```python
from build123d import *

# Parameters (mm, degrees)
F0_W      = 30
F0_H      = 50
F1_DEPTH  = 400
F3_D      = 20
F4_DEPTH  = 4.6
F5_W      = 10
F5_H      = 50
F6_DEPTH  = 20
F7_W      = 10
F7_H      = 25
F9_W      = 10
F9_H      = 25
F12_D     = 20
F13_W     = 30
F13_H     = 100
F14_DEPTH = 50
F16_D     = 10


with BuildPart() as f1:
    # F0 (on Front) → F1 (new body)
    with BuildSketch(Plane.XZ):
        with Locations((15, 25)):
            Rectangle(F0_W, F0_H)
    extrude(amount=F1_DEPTH)

    # F3 (through all)
    with Locations(Plane(origin=(0, 0, 0), x_dir=(0, 1, 0), z_dir=(-1, 0, 0))):
        with Locations((-375, -25), (-57.4, -25)):
            Hole(F3_D / 2)

    # F0 (on Front) → F4 (join)
    with BuildSketch(Plane.XZ):
        with Locations((15, 25)):
            Rectangle(F0_W, F0_H)
    extrude(amount=-F4_DEPTH)

    # F5 (on Right) → F6 (join)
    with BuildSketch(Plane.YZ):
        with Locations((-0.4, 25)):
            Rectangle(F5_W, F5_H)
        with Locations((-114.4, 25)):
            Rectangle(F5_W, F5_H)
    extrude(amount=-F6_DEPTH)

    # F7 (on face) → F8 (revolve)
    with BuildSketch(Plane(origin=(-20, 0, 0), x_dir=(0, -1, 0), z_dir=(-1, 0, 0))):
        with Locations((0.4, 12.5)):
            Rectangle(F7_W, F7_H)
    revolve(axis=Axis((-20, -0.4124408588, 25), (0, -1, 0)))

    # F9 (on face) → F10 (revolve)
    with BuildSketch(Plane(origin=(-20, 0, 0), x_dir=(0, -1, 0), z_dir=(-1, 0, 0))):
        with Locations((114.4, 12.5)):
            Rectangle(F9_W, F9_H)
    revolve(axis=Axis((-20, -114.0791960061, 25), (0, -1, 0)))

    # F12 (through all)
    with Locations(Plane(origin=(0, 4.6, 0), x_dir=(-1, 0, 0), z_dir=(0, 1, 0))):
        with Locations((20, 25)):
            Hole(F12_D / 2)

    # F13 (on face) → F14 (join)
    with BuildSketch(Plane(origin=(0, 0, 0), x_dir=(1, 0, 0), z_dir=(0, 0, -1))):
        with Locations((15, 57.4)):
            Rectangle(F13_W, F13_H)
    extrude(amount=F14_DEPTH)

    # F16 (through all)
    with Locations(Plane(origin=(0, 0, 0), x_dir=(0, -1, 0), z_dir=(-1, 0, 0))):
        with Locations((57.4, -35)):
            Hole(F16_D / 2)


solid = f1.part
```
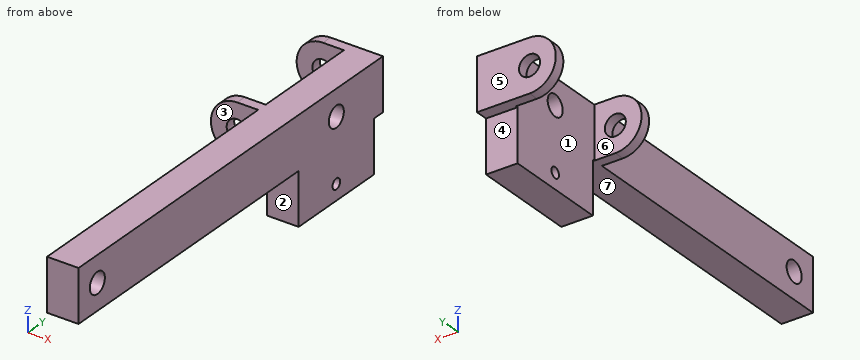
Input: part model. Units: mm. Frame: model coordinates. Face numbers are marked on the shaded views. A direction names the side the tool comes from. Give positions to 0.01 mm unless a question says otherwise; leave off trailing zeros. Order: outer loops, then holes, each group sorted by start corner. A loop starts at its lowest first (then second) coordinate and runs counter-clockwise, first axis right, second up.
1. Cut plane D-D (x = 10). Return loops of the section in (y, z).
Computed:
outline: (-400, 0) - (-107.4, 0) - (-107.4, -50) - (-7.4, -50) - (-7.4, 0) - (4.6, 0) - (4.6, 50) - (-400, 50) - close; hole circle Ø20 at (-375, 25); hole circle Ø20 at (-57.4, 25); hole circle Ø10 at (-57.4, -35)
2. Cut plane A-A (z = 25). Return loops of the section in (x, y), and give its area (3 significant figures).
Computed:
outline: (-45, -119.4) - (-30, -119.4) - (-30, -109.4) - (-45, -109.4) - close; (-45, -5.4) - (-30, -5.4) - (-30, 4.6) - (-45, 4.6) - close; (-10, -119.4) - (0, -119.4) - (0, -365) - (30, -365) - (30, -67.4) - (0, -67.4) - (0, -109.4) - (-10, -109.4) - close; (-10, -5.4) - (0, -5.4) - (0, -47.4) - (30, -47.4) - (30, 4.6) - (-10, 4.6) - close; (0, -400) - (30, -400) - (30, -385) - (0, -385) - close
area: 11,400 mm2
3. Cut plane C-C (z = -35). Return loops of the section in (x, y), and give its area (3 significant figures).
Computed:
outline: (0, -107.4) - (30, -107.4) - (30, -62.4) - (0, -62.4) - close; (0, -52.4) - (30, -52.4) - (30, -7.4) - (0, -7.4) - close
area: 2,700 mm2
4. Line query: probe 1 along Y at (x, z) = (-26.5, 12); probe 2 along X at (y, z) = (-84, -30); probe 3 along Y at (x, z) = (7, -23). Output: solid intervals per line, ascending.
Computed:
probe 1: y = -119.4 to -109.4, -5.4 to 4.6
probe 2: x = 0 to 30
probe 3: y = -107.4 to -7.4
5. Cut plane B-B (y = -375). Return loops of the section in (x, z), and give its area (3 significant figures).
Computed:
outline: (0, 0) - (30, 0) - (30, 15) - (0, 15) - close; (0, 35) - (30, 35) - (30, 50) - (0, 50) - close
area: 900 mm2
6. Set-up query: the marked faces 1, 2, 3 and 4. Return all of +Z, -Z, +X, -X, +Y, -Y with unobstructed straight access to the full face (end or side cutting, diameter ignored); none if empty.
Computed:
face 1: +Z, -Z, -X
face 2: -Z, +X, -X, -Y
face 3: +Z, -Z, -X, -Y
face 4: -Z, +X, -X, +Y
7. Pin query (flat end, axial travel): pin 1 Ø24 at (x, z) = (10, -32) entering from -Y; pin 2 Ø6 at (x, y) = (21, -199) entering from -Z; pin 3 Ø12 at (x, z) = (-20, 25) entering from -Y; pin 4 Ø6 at (y, z) = (-90, -6) entering from -X. Return the tip coordinate at first contact, or that it passes through.
Computed:
pin 1: stops at y = -107.4
pin 2: stops at z = 0
pin 3: passes through
pin 4: stops at x = 0
8. Draft query along Y for the marked faces 5, 6 and 7. Return one class per face: released by +Y, released by -Y, zero draft, split by the parting line, or undercut.
Computed:
face 5: released by +Y
face 6: undercut
face 7: zero draft
